Autodesk Inventor part; units mm, degrees
ref_plane "YZ Plane" through (0, 0, 0) normal (1, 0, 0) x (0, 1, 0)
ref_plane "XZ Plane" through (0, 0, 0) normal (0, 1, 0) x (-1, 0, 0)
ref_plane "XY Plane" through (0, 0, 0) normal (0, 0, 1) x (1, 0, 0)
sketch "Sketch1" plane through (0, 0, 0) normal (0, 0, 1) x (1, 0, 0)
  line L0 (0, 0) -> (27, 0)
  line L1 (27, 0) -> (27, 6.35)
  line L2 (27, 6.35) -> (0, 6.35)
  line L3 (0, 6.35) -> (0, 0)
  line L4 (0, 0) -> (0, -5)
  line L5 (0, -5) -> (3.5, -5)
  line L6 (3.5, -5) -> (3.5, 0)
  line L7 (27, 0) -> (27, -5)
  line L8 (27, -5) -> (23.5, -5)
  line L9 (23.5, -5) -> (23.5, 0)
  dimension "d0" = 27
  dimension "d1" = 6.35
  dimension "d14" = 20
  dimension "d15" = 5
extrude "Extrusion1" add sketch "Sketch1" along normal blind 12
sketch "Sketch2" plane through (0, 6.35, 0) normal (0, 1, 0) x (1, 0, 0)
  line L0 (0, 0) -> (0, -12)
  line L1 (27, 0) -> (27, -12)
  point P0 (6.5, -6)
  point P1 (20.5, -6)
  point P2 (0, -6)
  dimension "d4" = 6.5
  dimension "d5" = 6.5
  dimension "d6" = 14
hole "Hole1" at (6.5, 6.35, 6) at (20.5, 6.35, 6) direction (0, -1, 0) diameter 5 end through all
sketch "Sketch3" plane through (3.5, 0, 0) normal (0, -1, 0) x (1, 0, 0)
  circle A0 centre (3, 6) radius 2.5
  circle A1 centre (17, 6) radius 2.5
  line L0 (0, 0) -> (20, 0)
  line L1 (20, 0) -> (20, 12)
  line L2 (0, 12) -> (20, 12)
  line L3 (0, 0) -> (0, 12)
  line L4 (7.7343, 6) -> (5.3671, 1.9)
  line L5 (5.3671, 1.9) -> (0.6329, 1.9)
  line L6 (0.6329, 1.9) -> (-1.7343, 6)
  line L7 (-1.7343, 6) -> (0.6329, 10.1)
  line L8 (0.6329, 10.1) -> (5.3671, 10.1)
  line L9 (5.3671, 10.1) -> (7.7343, 6)
  point P0 (-3.5, 0)
  point P1 (0, 9.0038)
  point P2 (0, 2.9962)
  dimension "d16" = 8.2
extrude "Extrusion2" cut sketch "Sketch3" along normal blind 6.75 and the other way blind 3.5 contours L6 L7 L3 | L3 L7 L8 L9 L4 L5 L6
ref_plane "Work Plane1" through (13.5, -5, 0) normal (1, 0, 0) x (0, 0, -1)
mirror "Mirror1" about plane through (13.5, -5, 0) normal (1, 0, 0) of "Extrusion2"
properties part number "Idle Bearing mount"
Design review of the part built by this model. Coordinates are the model's own, in mm. A direction names the side the tool comes from. Give positions to 0.01 mm unless a question says otherwise; leave off trailing zeros. Order: outer loops, then holes, each group sorted by start corner. A loop starts at its lowest first (then second) coordinate and runs counter-clockwise, first axis right, second up. Notation, with made-up numbers: (5, -25.75) - (64, -25.75) arc R19 ccw to (64, 5.25) - close; hole circle Ø3 at (19.25, -30). An arc over 180 degrees is marked (long way). Use a Markdown table: item, result. Add a question column.
(1) Add section A-A on y = -2.25. Give the boundary of the cut face in (x, z).
(2) Wall thickness on probe 1 along X at (y, z) = (5.4, 6); probe 2 along Z at (x, y) = (20.5, 5.3); probe 3 along X at (y, z) = (5.75, 7): over which ranges is each line inside the solid? List them lowest first. Write a range as [from, to].
(3) Mouldability with a two-part tool opening along Y and no side actions: class faces 1 (the face through (9, 3.5, 8)), 2 (the face through (7, 2, 1.9)) as +Y half, -Y half, draft (parallel to the pull), parting line (faces both ways), or undercut.
(4) Machinability: for faces 3 (the face through (3.5, -3, 10)), 4 (the face through (5.749, 4.905, 8.385)), 5 (the face through (24.07, -0.69, 3.98)), which of the approach directions +Z, -Z, +X, -X, +Y, -Y give a long, thin tool a straight path to every point of the face, cutting with its end or side? Answer none if there is none.
(5) Clearance check with flat-ended pins moving along their axes: P1, Ø6.5, axis at x = 20.5, z = 6.5, coming from the -Y side; P2, Ø6, axis at x = 8, z = 9, coming from the -Y side; P3, Ø3, axis at x = 6.5, z = 6, coming from the +Y side. State where each tip first meets the part, or that it passes through.
(6) Add section D-D on y = 5.5. Give the boundary of the cut face in (x, z).
(7) Add section B-B on x = 8.5. Give the boundary of the cut face in (y, z).
(8) Add section C-C on z = 7. Give the boundary of the cut face in (x, y), then the cut area to 3 significant figures.
Report:
| question | item | result |
|---|---|---|
| 1 | outline | (0, 0) - (3.5, 0) - (3.5, 3) - (1.77, 6) - (3.5, 9) - (3.5, 12) - (0, 12) - close; (23.5, 0) - (27, 0) - (27, 12) - (23.5, 12) - (23.5, 9) - (25.23, 6) - (23.5, 3) - close |
| 2 | probe 1 | x = [0, 4], [9, 18], [23, 27] |
| 2 | probe 2 | z = [0, 3.5], [8.5, 12] |
| 2 | probe 3 | x = [0, 4.21], [8.79, 18.21], [22.79, 27] |
| 3 | face 1 | -Y half |
| 3 | face 2 | draft |
| 4 | face 3 | +Z, -Z, -Y |
| 4 | face 4 | +Y, -Y |
| 4 | face 5 | -Y |
| 5 | P1 | stops at y = 3.5 |
| 5 | P2 | stops at y = 0 |
| 5 | P3 | passes through |
| 6 | outline | (0, 0) - (27, 0) - (27, 12) - (0, 12) - close; hole circle Ø5 at (6.5, 6); hole circle Ø5 at (20.5, 6) |
| 7 | outline | (0, 0) - (6.35, 0) - (6.35, 4.5) - (3.5, 4.5) - (3.5, 1.9) - (0, 1.9) - close; (0, 10.1) - (3.5, 10.1) - (3.5, 7.5) - (6.35, 7.5) - (6.35, 12) - (0, 12) - close |
| 8 | outline | (0, -5) - (2.34, -5) - (2.34, 3.5) - (4.21, 3.5) - (4.21, 6.35) - (0, 6.35) - close; (8.79, 3.5) - (10.66, 3.5) - (10.66, 0) - (16.34, 0) - (16.34, 3.5) - (18.21, 3.5) - (18.21, 6.35) - (8.79, 6.35) - close; (22.79, 3.5) - (24.66, 3.5) - (24.66, -5) - (27, -5) - (27, 6.35) - (22.79, 6.35) - close |
| 8 | area | 111 mm² |
